```python
from build123d import *

# Parameters (mm, degrees)
BOSS_EXTRUDE1_DEPTH      = 10
BOSS_EXTRUDE1_DEPTH_BACK = 10
SKETCH2_R                = 7.5


with BuildPart() as part:
    # Sketch1 → Boss-Extrude1 (new, two sides)
    with BuildSketch(Plane.XY) as boss_extrude1_sk:
        Polygon((0, 0), (100, 0), (100, 45), (125, 45), (125, 100), (25, 100), (25, 55), (0, 55), align=None)
    extrude(amount=BOSS_EXTRUDE1_DEPTH)
    extrude(boss_extrude1_sk.sketch, amount=-BOSS_EXTRUDE1_DEPTH_BACK)

    # Sketch2 → Cut-Revolve2 (revolve, cut)
    with BuildSketch(Plane.XY):
        with Locations((82.5, 50)):
            Circle(SKETCH2_R)
    revolve(axis=Axis((62.5, 50.212189842, 0), (0, -1, 0)), mode=Mode.SUBTRACT)


solid = part.part
```
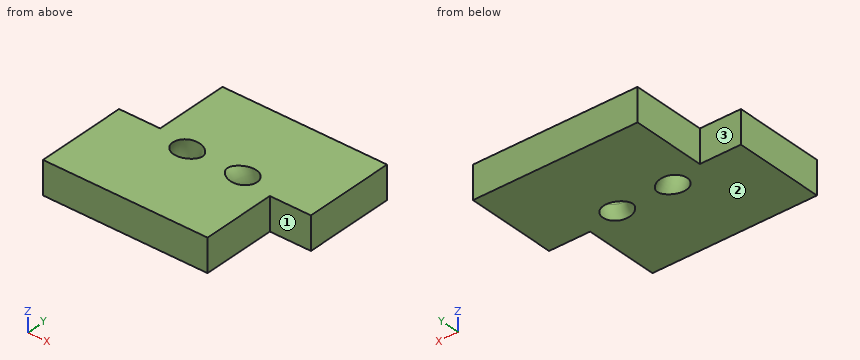
The model under review builds one solid part; all positions refer to its coordinate system, in mm. Face numbers are marked on the shaded views. A direction names the side the tool comes from. Round coordinates to 2 decimals unless told otherwise and drop trailing zeros. Loops run counter-clockwise (first coordinate to the right, second up) from the corner with the lowest first, then second, coordinate; pieces in that order, holes last. Notation, with made-up numbers: (1.5, 85) -> (18.5, 85) arc R14 cw to (18.5, 111) -> close; hole circle Ø9 at (-29, 9). An arc over 180 degrees is marked (long way). Answer in a Markdown table with one row per item.
1) Wall thickness on line 1 along X through (y, z) = (81, 7.5); line 2 along X through (y, z) = (29.5, 8.25); line 3 along Y through (x, z) = (24, 8): over which ranges is each line inside the solid? List them lowest first.
Taken from the geometry:
| item | result |
|---|---|
| line 1 | x = 25 to 125 |
| line 2 | x = 0 to 100 |
| line 3 | y = 0 to 55 |
2) Consider section B-B, the plane x = 103.5. Write out the cut boundary in (y, z).
Taken from the geometry:
| item | result |
|---|---|
| outline | (45, -10) -> (100, -10) -> (100, 10) -> (45, 10) -> close |
3) Consider section C-C, the plane y = 70.5. Write out the cut boundary in (x, z), plus the area to 3 significant figures.
Taken from the geometry:
| item | result |
|---|---|
| outline | (25, -10) -> (125, -10) -> (125, 10) -> (25, 10) -> close |
| area | 2,000 mm² |
4) For pin 1 Ø5 at (x, z) = (56, -3) entering from -Y; pin 2 Ø6 at (y, z) = (18.5, -4) entering from +X; pin 3 Ø3 at (x, z) = (107.5, -2) entering from -Y; pin 4 Ø10 at (y, z) = (84, 2.5) entering from -X, all flat-tipped, find the tip position at first contact; note any pin that passes through.
Taken from the geometry:
| item | result |
|---|---|
| pin 1 | stops at y = 0 |
| pin 2 | stops at x = 100 |
| pin 3 | stops at y = 45 |
| pin 4 | stops at x = 25 |
5) Consider section A-A, the plane z = 5.5. Count the separate pieces of the cut face and the enclosed holes in it, plus the area to 3 significant figures.
Taken from the geometry:
| item | result |
|---|---|
| separate pieces | 1 |
| enclosed holes | 2 |
| area | 9,880 mm² |
6) Tool access review of the marked faces 1, 2 and 3: name each direction out of +Z, -Z, +X, -X, +Y, -Y from which nothing blocks a thin tool from reaching the whole face with its end or side.
Taken from the geometry:
| item | result |
|---|---|
| face 1 | +Z, -Z, +X, -Y |
| face 2 | -Z, +X, -X, +Y, -Y |
| face 3 | +Z, -Z, -X, +Y |
